Input: part model. Units: mm. Frame: model coordinates. A direction names the side the tool comes from. Round coordinates to 2 decimals unless told otherwise and drop trailing zeros. Loops run counter-clockwise (first coordinate to the right, second up) from the corner with the lowest first, then second, coordinate; pieces in that order, holes last.
(1) Access query for faces 4 (the face through (4, 5, 400)), 5 (the face through (-8, -17, 197)). Directions: +Z, -Z, +X, -X, +Y, -Y. A direction counts if a zero-diameter tool reaches every point of the face in a straight line with its end or side. Return the directions, or none.
(2) Cut plane A-A, the plane x = 0. Output: boundary loops of the cut face in (y, z).
(3) Line query: line 1 (Y direction, x = 0, z = 82.5); line 2 (Y direction, x = -9.5, z = 153.5); line 3 (X direction, y = 10, z = 228). Output: solid intervals per line, ascending.
(4) Draft query along X for faces 1 (the face through (-17, -9, 197)), 2 (the face through (-11, 20, 197)), 3 (the face through (20, 11, 197)). Return one class per face: released by +X, released by -X, zero draft, split by the parting line, or undercut.
(5) First-contact query: pin 1 Ø3.5 at (x, z) = (-19, 292) entering from +Y; pin 2 Ø1.5 at (x, z) = (3.5, 135) entering from -Y; pin 3 Ø2.5 at (y, z) = (18.5, 222.5) entering from -X. Flat tips, straight axial feed; report the tip coordinate or a pass-through.
from build123d import *

# Parameters (mm, degrees)
F0_R     = 5
F1_DEPTH = 400


with BuildPart() as f1:
    # F0 (on Top) → F1 (new body)
    with BuildSketch(Plane.XY):
        with BuildLine():
            ThreePointArc((20, 17), (19.12132, 19.12132), (17, 20))
            Line((17, 20), (5, 20))
            Line((5, 20), (5, 17))
            Line((5, 17), (12, 17))
            Line((12, 17), (12, 14))
            Line((12, 14), (6, 8))
            Line((6, 8), (0, 8))
            Line((0, 8), (-6, 8))
            Line((-6, 8), (-12, 14))
            Line((-12, 14), (-12, 17))
            Line((-12, 17), (-5, 17))
            Line((-5, 17), (-5, 20))
            Line((-5, 20), (-17, 20))
            ThreePointArc((-17, 20), (-19.12132, 19.12132), (-20, 17))
            Line((-20, 17), (-20, 5))
            Line((-20, 5), (-17, 5))
            Line((-17, 5), (-17, 12))
            Line((-17, 12), (-14, 12))
            Line((-14, 12), (-8, 6))
            Line((-8, 6), (-8, 0))
            Line((-8, 0), (-8, -6))
            Line((-8, -6), (-14, -12))
            Line((-14, -12), (-17, -12))
            Line((-17, -12), (-17, -5))
            Line((-17, -5), (-20, -5))
            Line((-20, -5), (-20, -17))
            ThreePointArc((-20, -17), (-19.12132, -19.12132), (-17, -20))
            Line((-17, -20), (-5, -20))
            Line((-5, -20), (-5, -17))
            Line((-5, -17), (-12, -17))
            Line((-12, -17), (-12, -14))
            Line((-12, -14), (-6, -8))
            Line((-6, -8), (0, -8))
            Line((0, -8), (6, -8))
            Line((6, -8), (12, -14))
            Line((12, -14), (12, -17))
            Line((12, -17), (5, -17))
            Line((5, -17), (5, -20))
            Line((5, -20), (17, -20))
            ThreePointArc((17, -20), (19.12132, -19.12132), (20, -17))
            Line((20, -17), (20, -5))
            Line((20, -5), (17, -5))
            Line((17, -5), (17, -12))
            Line((17, -12), (14, -12))
            Line((14, -12), (8, -6))
            Line((8, -6), (8, 0))
            Line((8, 0), (8, 6))
            Line((8, 6), (14, 12))
            Line((14, 12), (17, 12))
            Line((17, 12), (17, 5))
            Line((17, 5), (20, 5))
            Line((20, 5), (20, 17))
        make_face()
        Circle(F0_R, mode=Mode.SUBTRACT)
    extrude(amount=F1_DEPTH)


solid = f1.part
Reported:
1. face 4: +Z, +X, -X, +Y, -Y
1. face 5: +Z, -Z
2. outline: (-8, 0) - (-5, 0) - (-5, 400) - (-8, 400) - close; (5, 0) - (8, 0) - (8, 400) - (5, 400) - close
3. line 1: y = -8 to -5, 5 to 8
3. line 2: y = -20 to -17, -11.5 to -7.5, 7.5 to 11.5, 17 to 20
3. line 3: x = -20 to -17, -12 to -8, 8 to 12, 17 to 20
4. face 1: undercut
4. face 2: zero draft
4. face 3: released by +X
5. pin 1: stops at y = 19.99
5. pin 2: stops at y = -8
5. pin 3: stops at x = -19.99
